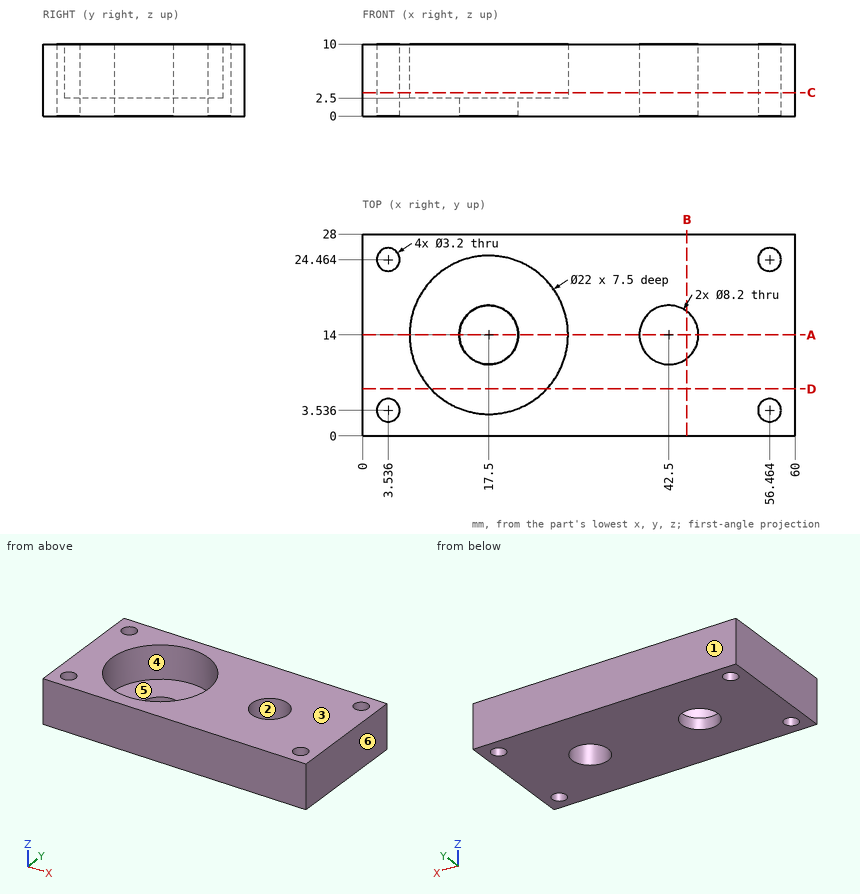
Can you work these out from the drawing? Everything is in mm from the part's minimum corner. A direction names the side the tool comes from. Coordinates: 2 decimals unless noted, no trailing zeros. Loops run counter-clockwise (first coordinate to the right, second up) from the corner with the lowest first, then second, coordinate; pieces in that order, holes last. Notation, with made-up numbers: (57.25, 58.5) - (76.25, 58.5) arc R23 cw to (76.25, 84.5) - close; hole circle Ø9 at (-23.75, -21). An arc over 180 degrees is marked (long way). Put each result on its own line as item: value. Start each with the question number.
Item 1: Suppose I cut it at A-A (y = 14). Please give me the cut outline in (x, z).
Item 2: If we mould it in two halves opening along Y, with no side actions, what happens to the marked faces 1, 2, 3 and 4? For each: +Y half, -Y half, draft (parallel to the pull), parting line (faces both ways), or undercut.
Item 3: Which directions (+Z, -Z, +X, -X, +Y, -Y) give clear straight access to the entire face, cutting with the end or side of a thin tool? Please do the marked faces 5 and 6.
Item 4: For pin 1 (13 mm diameter, centred on x = 17.5, y = 14, fed in from +Z); pin 2 (1.9 mm diameter, centred on x = 3.54, y = 3.54, fed in from -Z), each with a flat end and sliding along its axis, tell me the tip position at first contact or that it passes through.
Item 5: Suppose I cut it at D-D (y = 6.5). Please give me the cut outline in (x, z), and give its area (3 significant figures).
Item 6: Suppose I cut it at C-C (z = 3.25). Please give me the cut outline in (x, y) (1 decimal).
Item 7: If I drill on line 1 along X through (y, z) = (13.75, 1.75); line 2 along X through (y, z) = (23.25, 1) (1 decimal); line 3 along Y through (x, z) = (42.5, 4.5), over which ranges is the centre line in solid material (lowest first)?
Item 8: Suppose I cut it at B-B (x = 45). Please give me the cut outline in (y, z), and give its area (3 significant figures).
Here are the results:
1. outline: (0, 0) - (13.4, 0) - (13.4, 2.5) - (6.5, 2.5) - (6.5, 10) - (0, 10) - close; (21.6, 0) - (38.4, 0) - (38.4, 10) - (28.5, 10) - (28.5, 2.5) - (21.6, 2.5) - close; (46.6, 0) - (60, 0) - (60, 10) - (46.6, 10) - close
2. face 1: +Y half
2. face 2: undercut
2. face 3: draft
2. face 4: undercut
3. face 5: +Z
3. face 6: +Z, -Z, +X, +Y, -Y
4. pin 1: z = 2.5
4. pin 2: through
5. outline: (0, 0) - (60, 0) - (60, 10) - (25.55, 10) - (25.55, 2.5) - (9.45, 2.5) - (9.45, 10) - (0, 10) - close
5. area: 479 mm²
6. outline: (0, 0) - (60, 0) - (60, 28) - (0, 28) - close; hole circle Ø3.2 at (3.5, 3.5); hole circle Ø3.2 at (3.5, 24.5); hole circle Ø22 at (17.5, 14); hole circle Ø8.2 at (42.5, 14); hole circle Ø3.2 at (56.5, 3.5); hole circle Ø3.2 at (56.5, 24.5)
7. line 1: 0 to 13.41, 21.59 to 38.41, 46.59 to 60
7. line 2: 0 to 2.5, 4.6 to 55.4, 57.5 to 60
7. line 3: 0 to 9.9, 18.1 to 28
8. outline: (0, 0) - (10.75, 0) - (10.75, 10) - (0, 10) - close; (17.25, 0) - (28, 0) - (28, 10) - (17.25, 10) - close
8. area: 215 mm²
